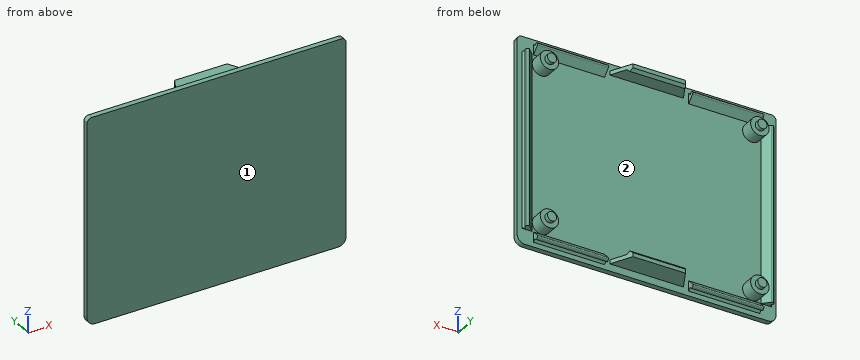
```python
from build123d import *

# Parameters (mm, degrees)
SKETCH2_R            = 3.5
BOSS_EXTRUDE1_DEPTH  = 5
SKETCH3_R            = 1.75
BOSS_EXTRUDE2_DEPTH  = 1.6
SKETCH1_W            = 98.44
SKETCH1_H            = 78.44
BOSS_EXTRUDE4_DEPTH  = 2
BOSS_EXTRUDE5_START  = -63.5
BOSS_EXTRUDE5_DEPTH  = 67
FILLET1_R            = 0.5
FILLET1_OF_MIRROR1_R = 0.5
BOSS_EXTRUDE8_DEPTH  = 43
CUT_EXTRUDE4_DEPTH   = 16
BOSS_EXTRUDE9_DEPTH  = 14
CHAMFER3_START       = -66.5
CHAMFER3_DEPTH       = 2.5
CHAMFER4_SIZE2       = 4
CHAMFER4_SIZE        = 7.8
FILLET2_R            = 0.5
FILLET2_OF_MIRROR2_R = 0.5
FILLET3_R            = 3
CHAMFER5_SIZE2       = 4
CHAMFER5_SIZE        = 7.8
CHAMFER6_SIZE2       = 7.8
CHAMFER6_SIZE        = 4
FILLET4_R            = 1.8


with BuildPart() as part:
    # Sketch2 → Boss-Extrude1 (new body)
    with BuildSketch(Plane(origin=(0, 0, 0), x_dir=(1, 0, 0), z_dir=(0, 1, 0))):
        with Locations(Location((0, 0, 0), (0, 0, 270))):
            Circle(SKETCH2_R)
    boss_extrude1 = extrude(amount=BOSS_EXTRUDE1_DEPTH)

    # Sketch3 → Boss-Extrude2 (add)
    with BuildSketch(Plane(origin=(0, 5, 0), x_dir=(1, 0, 0), z_dir=(0, 1, 0))):
        with Locations(Location((0, 0, 0), (0, 0, 270))):
            Circle(SKETCH3_R)
    boss_extrude2 = extrude(amount=BOSS_EXTRUDE2_DEPTH)

    # Sketch1 → Boss-Extrude4 (add)
    with BuildSketch(Plane(origin=(0, 0, 0), x_dir=(1, 0, 0), z_dir=(0, 1, 0))):
        with Locations((40, 30)):
            Rectangle(SKETCH1_W, SKETCH1_H)
    extrude(amount=-BOSS_EXTRUDE4_DEPTH)

    # Sketch-Pattern2: Boss-Extrude1, Boss-Extrude2 at 3 more places
    with Locations((80, 0, 0), (80, 0, -60), (0, 0, -60)):
        add(boss_extrude1)
        add(boss_extrude2)

    # Sketch6 → Boss-Extrude5 (add)
    with BuildSketch(Plane.XY.offset(BOSS_EXTRUDE5_START)):
        Polygon((-7.421320344, 1.8), (-6.360660172, 2.860660172), (-3.5, 0), (-7.421320344, 0), (-6.521320344, 0.9), align=None)
    boss_extrude5 = extrude(amount=BOSS_EXTRUDE5_DEPTH)

    # Fillet1
    fillet1_edges = [part.edges().sort_by_distance(p)[0] for p in [
        (-7.421320344, 1.8, -30),
        (-6.360660172, 2.860660172, -30),
    ]]
    fillet(fillet1_edges, radius=FILLET1_R)

    # Mirror1: Boss-Extrude5 across plane
    add(boss_extrude5.mirror(Plane(origin=(40, 0, 0), x_dir=(0, 0, 1), z_dir=(1, 0, 0))))

    # Fillet1 of Mirror1
    fillet1_of_mirror1_edges = [part.edges().sort_by_distance(p)[0] for p in [
        (87.421320344, 1.8, -30),
        (86.360660172, 2.860660172, -30),
    ]]
    fillet(fillet1_of_mirror1_edges, radius=FILLET1_OF_MIRROR1_R)

    # Sketch8 → Boss-Extrude8 (add, symmetric)
    with BuildSketch(Plane(origin=(40, 0, 0), x_dir=(0, 0, -1), z_dir=(1, 0, 0))):
        Polygon((66.360660172, 2.860660172), (63.5, 0), (67.421320344, 0), (66.521320344, 0.9), (67.421320344, 1.8), align=None)
    boss_extrude8 = extrude(amount=BOSS_EXTRUDE8_DEPTH, both=True)

    # Sketch8<4> → Cut-Extrude4 (cut, symmetric)
    with BuildSketch(Plane(origin=(40, 0, 0), x_dir=(0, 0, -1), z_dir=(1, 0, 0))):
        Polygon((66.360660172, 2.860660172), (63.5, 0), (67.421320344, 0), (66.521320344, 0.9), (67.421320344, 1.8), align=None)
    cut_extrude4 = extrude(amount=CUT_EXTRUDE4_DEPTH, both=True, mode=Mode.SUBTRACT)

    # Sketch7 → Boss-Extrude9 (add, symmetric)
    with BuildSketch(Plane(origin=(40, 0, 0), x_dir=(0, 0, -1), z_dir=(1, 0, 0))):
        Polygon((66.5, 7.8), (66.5, 0), (65, 0), (65, 5.8), (64, 6.8), (65, 7.8), align=None)
    boss_extrude9 = extrude(amount=BOSS_EXTRUDE9_DEPTH, both=True)

    # Chamfer3: read off the stored shape, not the designer's step
    # Chamfer3 outline → Chamfer3 (cut)
    with BuildSketch(Plane.XY.offset(CHAMFER3_START)):
        Polygon((26, 7.8), (26, 0), (30, 7.8), align=None)
    extrude(amount=CHAMFER3_DEPTH, mode=Mode.SUBTRACT)

    # Chamfer4
    chamfer4_edges = [part.edges().sort_by_distance(p)[0] for p in [
        (54, 7.8, -65.75),
    ]]
    chamfer4_side = [part.faces().sort_by_distance(p)[0] for p in [
        (54, 7.72, -65.75),
    ]]
    chamfer(chamfer4_edges, length=CHAMFER4_SIZE - 0.0001, length2=CHAMFER4_SIZE2 - 0.0001, reference=chamfer4_side[0])  # a hair under: the kernel refuses the full size

    # Fillet2
    fillet2_edges = [part.edges().sort_by_distance(p)[0] for p in [
        (10.5, 2.860660172, -66.360660172),
        (10.5, 1.8, -67.421320344),
        (69.5, 2.860660172, -66.360660172),
        (69.5, 1.8, -67.421320344),
    ]]
    fillet(fillet2_edges, radius=FILLET2_R)

    # Mirror2: Boss-Extrude8, Cut-Extrude4 across plane
    add(boss_extrude8.mirror(Plane.XY.offset(-30)))
    add(cut_extrude4.mirror(Plane.XY.offset(-30)), mode=Mode.SUBTRACT)

    # Fillet2 of Mirror2
    fillet2_of_mirror2_edges = [part.edges().sort_by_distance(p)[0] for p in [
        (10.5, 2.860660172, 6.360660172),
        (10.5, 1.8, 7.421320344),
        (69.5, 2.860660172, 6.360660172),
        (69.5, 1.8, 7.421320344),
    ]]
    fillet(fillet2_of_mirror2_edges, radius=FILLET2_OF_MIRROR2_R)

    # Fillet3
    fillet3_edges = [part.edges().sort_by_distance(p)[0] for p in [
        (-9.22, -1, -69.22),
        (89.22, -1, -69.22),
    ]]
    fillet(fillet3_edges, radius=FILLET3_R)

    # Mirror4: Boss-Extrude9 across plane
    add(boss_extrude9.mirror(Plane.XY.offset(-30)))

    # Chamfer5
    chamfer5_edges = [part.edges().sort_by_distance(p)[0] for p in [
        (26, 7.8, 5.75),
    ]]
    chamfer5_side = [part.faces().sort_by_distance(p)[0] for p in [
        (26, 7.72, 5.75),
    ]]
    chamfer(chamfer5_edges, length=CHAMFER5_SIZE - 0.0001, length2=CHAMFER5_SIZE2 - 0.0001, reference=chamfer5_side[0])  # a hair under: the kernel refuses the full size

    # Chamfer6
    chamfer6_edges = [part.edges().sort_by_distance(p)[0] for p in [
        (54, 7.8, 5.75),
    ]]
    chamfer6_side = [part.faces().sort_by_distance(p)[0] for p in [
        (53.92, 7.8, 5.75),
    ]]
    chamfer(chamfer6_edges, length=CHAMFER6_SIZE - 0.0001, length2=CHAMFER6_SIZE2 - 0.0001, reference=chamfer6_side[0])  # a hair under: the kernel refuses the full size

    # Fillet4
    fillet4_edges = [part.edges().sort_by_distance(p)[0] for p in [
        (89.22, -1, 9.22),
        (-9.22, -1, 9.22),
    ]]
    fillet(fillet4_edges, radius=FILLET4_R)


solid = part.part
```
CAD build for the part. Positions are in the model's coordinates, mm. Face numbers are marked on the shaded views. Round coordinates to 2 decimals unless told otherwise and drop trailing zeros. Write each loop counter-clockwise with the first axis right and the second up, starting at its lowest first coordinate (ties: lowest second). Pieces come first, ordered by that corner, then holes. Notation, with made-up numbers: (50.5, -16.5) -> (78.5, -16.5) arc R23 cw to (78.5, 21.5) -> close; hole circle Ø8 at (80, 19.25). An arc over 180 degrees is marked (long way). Answer in a Markdown table with one row per item. Add a question column.
Item 1: Saw through at B-B, the plane z = -48. Write the cut outline in (x, y), then the cut area to 3 significant figures.
Item 2: Saw through at A-A, the plane x = 20.5. Write the cut outline in (y, z).
Item 3: Saw through at C-C, the plane x = 38.5. Write the cut outline in (y, z), then the cut area to 3 significant figures.
Item 4: Drop flat-ended pins along their axis: pin 1 Ø1.8 at (x, z) = (80.5, -59.5) entering from +Y; pin 2 Ø12 at (x, z) = (7.5, -54.5) entering from +Y; pin 3 Ø0.8 at (y, z) = (1, 5) entering from -X; pin 4 Ø2 at (y, z) = (5, -46) entering from +X. Give the stop position or say it passes through.
Item 5: Mould opens along Z. For the marked faces 1 and 2 say: pulls with the +Z half, pulls with the -Z half, needs draft (parallel to the pull), parting line crosses it, or undercut.
Item 6: Drill centre lines: line 1 (X direction, y = 0.75, z = -59); line 2 (Z direction, x = 27, y = 0.75); line 3 (Z direction, x = 72.5, y = 2.5). Where is each one in solid material? Low to high. Write a range as from..to.
Findings below:
| question | item | result |
|---|---|---|
| 1 | outline | (-9.22, -2) -> (89.22, -2) -> (89.22, 0) -> (87.42, 0) -> (86.52, 0.9) -> (87.07, 1.45) arc R0.5 ccw to (87.07, 2.15) -> (86.71, 2.51) arc R0.5 ccw to (86.01, 2.51) -> (83.5, 0) -> (-3.5, 0) -> (-6.01, 2.51) arc R0.5 ccw to (-6.71, 2.51) -> (-7.07, 2.15) arc R0.5 ccw to (-7.07, 1.45) -> (-6.52, 0.9) -> (-7.42, 0) -> (-9.22, 0) -> close |
| 1 | area | 208 mm^2 |
| 2 | outline | (-2, -69.22) -> (0, -69.22) -> (0, -67.42) -> (0.9, -66.52) -> (1.45, -67.07) arc R0.5 ccw to (2.15, -67.07) -> (2.51, -66.71) arc R0.5 ccw to (2.51, -66.01) -> (0, -63.5) -> (0, 3.5) -> (2.51, 6.01) arc R0.5 ccw to (2.51, 6.71) -> (2.15, 7.07) arc R0.5 ccw to (1.45, 7.07) -> (0.9, 6.52) -> (0, 7.42) -> (0, 9.22) -> (-2, 9.22) -> close |
| 3 | outline | (-2, -69.22) -> (0, -69.22) -> (0, -66.5) -> (7.8, -66.5) -> (7.8, -65) -> (6.8, -64) -> (5.8, -65) -> (0, -65) -> (0, 5) -> (5.8, 5) -> (6.8, 4) -> (7.8, 5) -> (7.8, 6.5) -> (0, 6.5) -> (0, 9.22) -> (-2, 9.22) -> close |
| 3 | area | 182 mm^2 |
| 4 | pin 1 | stops at y = 6.6 |
| 4 | pin 2 | stops at y = 5 |
| 4 | pin 3 | stops at x = -3 |
| 4 | pin 4 | passes through |
| 5 | face 1 | needs draft |
| 5 | face 2 | undercut |
| 6 | line 1 | x = -6.67..-4.25, -3.35..3.35, 76.65..83.35, 84.25..86.67 |
| 6 | line 2 | z = -66.5..-65, 5..6.5 |
| 6 | line 3 | z = -66.72..-66, 6..6.72 |
